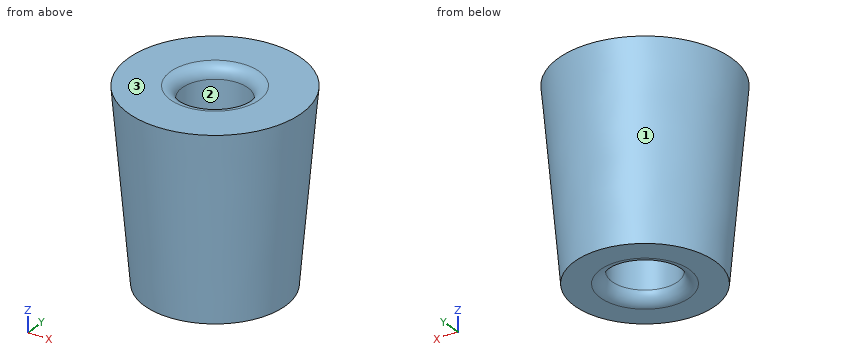
```python
from build123d import *

# Parameters (mm, degrees)
F0_R     = 6
F0_R_2   = 2.8
F1_DEPTH = 16
F1_TAPER = -5
F2_DEPTH = 16.0010001
F3_R     = 1


with BuildPart() as f1:
    # F0 (on Top) → F1 (new body)
    with BuildSketch(Plane.XY):
        Circle(F0_R)
        Circle(F0_R_2, mode=Mode.SUBTRACT)
    extrude(amount=F1_DEPTH, taper=F1_TAPER)

    # F0 (on Top) → F2 (cut, through all)
    with BuildSketch(Plane.XY):
        Circle(F0_R_2)
    extrude(amount=F2_DEPTH, mode=Mode.SUBTRACT)

    # F3
    f3_edges = [f1.edges().sort_by_distance(p)[0] for p in [
        (-2.8, 0, 16),
        (-2.8, 0, 0),
    ]]
    fillet(f3_edges, radius=F3_R)


solid = f1.part
```
Check sheet for the modelled part. Datum: model origin and axes. Units: mm. Face numbers are marked on the shaded views. Coordinates: 2 decimals unless noted, no trailing zeros. Order: outer loops, then holes, each group sorted by start corner. A loop starts at its lowest first (then second) coordinate and runs counter-clockwise, first axis right, second up. Notation, with made-up numbers: M 85.25,41 L 93.25,41 A29 ccw 93.25,63 Z; hole C 23.25,12 d11. An arc over 180 degrees is marked long. One line per question, with ' | ' between items. Start each with the question number.
Item 1: Mould release check, pull along X, two halves, no side actions. Record for the marked faces 1, 2 and 3: pulls with the +X half, pulls with the -X half, needs draft (parallel to the pull), parting line crosses it, or undercut.
Item 2: Gauge pin test, flat ends, axial feed: P1, Ø4, axis at x = 3.5, z = 12.5, coming from the +Y side; P2, Ø5, axis at x = 4.5, z = 9, coming from the +Y side; P3, Ø1, axis at x = -1, z = 7, coming from the -Y side. Record the tip position at first contact, or that the pin passes through.
Item 3: Material ranges on line 1 (X direction, y = -2, z = 4.5); line 2 (Y direction, x = 0, z = 8.25); line 3 (X direction, y = -0.75, z = 1.5), recorded low to high.
Item 4: Sectioned sample at C-C on z = 11.5. Record the cut outline in (x, y), and give its area (3 significant figures).
Item 5: Sectioned sample at A-A on x = 0. Record the cut outline in (y, z).
Item 6: Sectioned sample at B-B on z = 7.25. Record the cut outline in (x, y), and give its area (3 significant figures).
Answer below:
1) face 1: parting line crosses it | face 2: undercut | face 3: needs draft
2) P1: stops at y = 6.97 | P2: stops at y = 6.52 | P3: stops at y = -6.61
3) line 1: x = -6.07 to -1.96, 1.96 to 6.07 | line 2: y = -6.72 to -2.8, 2.8 to 6.72 | line 3: x = -6.09 to -2.7, 2.7 to 6.09
4) outline: C 0,0 d14.01; hole C 0,0 d5.6 | area: 130 mm^2
5) outline: M -7.4,16 L -6,0 L -3.8,0 A1 ccw -2.8,1 L -2.8,15 A1 ccw -3.8,16 Z; M 2.8,1 A1 ccw 3.8,0 L 6,0 L 7.4,16 L 3.8,16 A1 ccw 2.8,15 Z
6) outline: C 0,0 d13.27; hole C 0,0 d5.6 | area: 114 mm^2
